from build123d import *

# Parameters (mm, degrees)
BOSS_EXTRUDE1_DEPTH = 6
SKETCH4_R           = 2.5
SKETCH4_R_2         = 2
CUT_EXTRUDE1_DEPTH  = 6
CHAMFER1_SIZE       = 1.7
FILLET1_R           = 2
SKETCH5_R           = 4.25
CUT_EXTRUDE2_DEPTH  = 4


with BuildPart() as part:
    # Sketch1 → Boss-Extrude1 (new body)
    with BuildSketch(Plane(origin=(0, 0, 0), x_dir=(1, 0, 0), z_dir=(0, 1, 0))):
        with BuildLine():
            Line((-13.85, 5.29), (-13.85, -5.29))
            ThreePointArc((-13.85, -5.29), (-12.5791991, -11.085364527), (-9, -15.817226605))
            Line((-9, -15.817226605), (-9, -54.14))
            Line((-9, -54.14), (9, -54.14))
            Line((9, -54.14), (9, -15.817226605))
            ThreePointArc((9, -15.817226605), (12.5791991, -11.085364527), (13.85, -5.29))
            Line((13.85, -5.29), (13.85, 5.29))
            ThreePointArc((13.85, 5.29), (12.5791991, 11.085364527), (9, 15.817226605))
            Line((9, 15.817226605), (9, 54.14))
            Line((9, 54.14), (-9, 54.14))
            Line((-9, 54.14), (-9, 15.817226605))
            ThreePointArc((-9, 15.817226605), (-12.5791991, 11.085364527), (-13.85, 5.29))
        make_face()
    extrude(amount=BOSS_EXTRUDE1_DEPTH)

    # Sketch4 → Cut-Extrude1 (cut)
    with BuildSketch(Plane(origin=(0, 6, 0), x_dir=(1, 0, 0), z_dir=(0, 1, 0))):
        with Locations((0, 44.14)):
            Circle(SKETCH4_R)
        with Locations((0, -44.14)):
            Circle(SKETCH4_R)
        with Locations((-9.5, -5.29)):
            Circle(SKETCH4_R_2)
        with Locations((9.5, -5.29)):
            Circle(SKETCH4_R_2)
        with Locations((0, 4.21)):
            Circle(SKETCH4_R_2)
        with Locations((0, -14.79)):
            Circle(SKETCH4_R_2)
    extrude(amount=-CUT_EXTRUDE1_DEPTH, mode=Mode.SUBTRACT)

    # Chamfer1
    chamfer1_edges = [part.edges().sort_by_distance(p)[0] for p in [
        (-2, 6, 14.79),
        (-11.5, 6, 5.29),
        (7.5, 6, 5.29),
        (-2, 6, -4.21),
    ]]
    chamfer(chamfer1_edges, length=CHAMFER1_SIZE)

    # Fillet1
    fillet1_edges = [part.edges().sort_by_distance(p)[0] for p in [
        (9, 0, 34.978613303),
        (0, 0, 54.14),
        (-9, 0, 34.978613303),
        (-9, 0, -34.978613303),
        (0, 0, -54.14),
        (9, 0, -34.978613303),
    ]]
    fillet(fillet1_edges, radius=FILLET1_R)

    # Sketch5 → Cut-Extrude2 (cut)
    with BuildSketch(Plane.XZ):
        with Locations((0, -44.14)):
            Circle(SKETCH5_R)
        with Locations((0, 44.14)):
            Circle(SKETCH5_R)
    extrude(amount=-CUT_EXTRUDE2_DEPTH, mode=Mode.SUBTRACT)


solid = part.part
Work out the finished part from the listing and answer in its coordinate system (mm). A direction names the side the tool comes from. Give positions to 0.01 mm unless a question says otherwise; leave off trailing zeros. Loops run counter-clockwise (first coordinate to the right, second up) from the corner with the lowest first, then second, coordinate; pieces in that order, holes last. Notation, with made-up numbers: (40.5, -21) -> (95.5, -21) arc R8 cw to (95.5, -9) -> close; hole circle Ø9 at (-14, 1.25). An arc over 180 degrees is marked (long way). Use a Markdown table: item, result. Add a question column.
1. For faces 1 (the cylindrical face through (-0.553, 1.972, -39.926)), 2 (the flat face through (0, 4, -54.14)), 3 (the flat face through (-9, 4, -35)), 4 (the flat face through (9, 4, 35)), 5 (the cylindrical face through (-8.43, 0.6, 35.25)), determine the directions among +Z, -Z, +X, -X, +Y, -Y from which every point of the face is accessible in a straight line to the end or side of a thin tool.
2. Section A-A on z = -44.14 is taken. Determine the outline of the cut face in (x, y).
3. Section C-C on z = 31 is taken. Determine the outline of the cut face in (x, y).
4. Find the intervals of material crossed by probe 1 along X at (y, z) = (1.5, 5.29); probe 2 along Z at (x, y) = (0, 3.05); probe 3 along Z at (x, y) = (-0.5, 1.25), in increasing order.
5. Section B-B on z = -4.21 is taken. Determine the outline of the cut face in (x, y), and give its area (3 significant figures).
6. Flat-ended cylindrical pins translate along their axes: pin 1 Ø4 at (x, z) = (0, 44.14) entering from +Y; pin 2 Ø6.5 at (x, z) = (0, -4.21) entering from +Y; pin 3 Ø4.5 at (x, z) = (0, 14.79) entering from +Y; pin 4 Ø3 at (y, z) = (5, -26) entering from -X. Find the tip coordinate at first contact, or state that the pin passes through.
7. Determine the mould class of faces 6 (the cylindrical face through (8.43, 0.6, -35.25)), 7 (the flat face through (-9, 4, 35)), 8 (the cylindrical face through (-9.76, 2.18, 3.307)), 9 (the cylindrical face through (-0.54, 5.01, -41.7)) for opening direction X: released by +X, released by -X, zero draft, split by the parting line, or undercut.
Results below:
| question | item | result |
|---|---|---|
| 1 | face 1 | -Y |
| 1 | face 2 | -Z, +X, -X, +Y, -Y |
| 1 | face 3 | -Z, -X, +Y, -Y |
| 1 | face 4 | +Z, +X, +Y, -Y |
| 1 | face 5 | +Z, -X, -Y |
| 2 | outline | (-9, 2) arc R2 ccw to (-7, 0) -> (-4.25, 0) -> (-4.25, 4) -> (-2.5, 4) -> (-2.5, 6) -> (-9, 6) -> close; (2.5, 4) -> (4.25, 4) -> (4.25, 0) -> (7, 0) arc R2 ccw to (9, 2) -> (9, 6) -> (2.5, 6) -> close |
| 3 | outline | (-9, 2) arc R2 ccw to (-7, 0) -> (7, 0) arc R2 ccw to (9, 2) -> (9, 6) -> (-9, 6) -> close |
| 4 | probe 1 | x = -13.85 to -11.5, -7.5 to 7.5, 11.5 to 13.85 |
| 4 | probe 2 | z = -54.14 to -48.39, -39.89 to -6.21, -2.21 to 12.79, 16.79 to 39.89, 48.39 to 54.14 |
| 4 | probe 3 | z = -53.99 to -48.36, -39.92 to -6.15, -2.27 to 12.85, 16.73 to 39.92, 48.36 to 53.99 |
| 5 | outline | (-13.85, 0) -> (-2, 0) -> (-2, 4.3) -> (-3.7, 6) -> (-13.85, 6) -> close; (2, 0) -> (13.85, 0) -> (13.85, 6) -> (3.7, 6) -> (2, 4.3) -> close |
| 5 | area | 139 mm^2 |
| 6 | pin 1 | passes through |
| 6 | pin 2 | stops at y = 5.55 |
| 6 | pin 3 | stops at y = 4.55 |
| 6 | pin 4 | stops at x = -9 |
| 7 | face 6 | released by +X |
| 7 | face 7 | released by -X |
| 7 | face 8 | undercut |
| 7 | face 9 | undercut |
